```python
from build123d import *

# Parameters (mm, degrees)
F1_DEPTH = 25.4


with BuildPart() as f1:
    # F0 (on Front) → F1 (new body)
    with BuildSketch(Plane.XZ):
        with BuildLine():
            add(Edge.make_bspline(
                [(-41.275, 9.525), (-11.0804249201, 30.3606307657), (19.1141501598, 51.1962615313), (42.965290813, 58.9149246625)],
                knots=[0, 0, 0, 0, 0.5181088639, 0.5181088639, 0.5181088639, 0.5181088639], degree=3))
            Line((-41.275, 9.525), (22.225, 9.525))
            Line((22.225, 9.525), (22.225, 27.0002))
            ThreePointArc((22.225, 27.0002), (27.86556221, 46.0311571047), (42.965290813, 58.9149246625))
        make_face()
        Polygon((22.225, 9.525), (-41.275, 9.525), (-41.275, -9.525), (41.275, -9.525), (41.275, 9.525), align=None)
        with BuildLine():
            Line((22.225, 27.0002), (22.225, 9.525))
            Line((22.225, 9.525), (41.275, 9.525))
            Line((41.275, 9.525), (41.275, 27.0002))
            ThreePointArc((41.275, 27.0002), (45.9246798487, 38.2255201513), (57.15, 42.8752))
            Line((57.15, 42.8752), (60.325, 42.8752))
            Line((60.325, 42.8752), (60.325, 61.9252))
            Line((60.325, 61.9252), (57.15, 61.9252))
            add(Edge.make_bspline(
                [(42.965290813, 58.9149246625), (47.9955126784, 60.5427959923), (52.7435843005, 61.5872364295), (57.15, 61.9252)],
                knots=[0.5181088639, 0.5181088639, 0.5181088639, 0.5181088639, 0.6273783774, 0.6273783774, 0.6273783774, 0.6273783774], degree=3))
            ThreePointArc((42.965290813, 58.9149246625), (27.86556221, 46.0311571047), (22.225, 27.0002))
        make_face()
        with BuildLine():
            ThreePointArc((57.15, 61.9252), (49.8996942767, 61.1643433658), (42.965290813, 58.9149246625))
            add(Edge.make_bspline(
                [(42.965290813, 58.9149246625), (47.9955126784, 60.5427959923), (52.7435843005, 61.5872364295), (57.15, 61.9252)],
                knots=[0.5181088639, 0.5181088639, 0.5181088639, 0.5181088639, 0.6273783774, 0.6273783774, 0.6273783774, 0.6273783774], degree=3))
        make_face()
        with BuildLine():
            add(Edge.make_bspline(
                [(57.15, 61.9252), (58.2283036755, 62.0079038085), (59.2861476071, 62.0483009137), (60.325, 62.0494272736)],
                knots=[0.6273783774, 0.6273783774, 0.6273783774, 0.6273783774, 0.6541179604, 0.6541179604, 0.6541179604, 0.6541179604], degree=3))
            Line((57.15, 61.9252), (60.325, 61.9252))
            Line((60.325, 61.9252), (60.325, 62.0494272736))
        make_face()
        with BuildLine():
            Line((63.5542024739, 61.9252), (60.325, 61.9252))
            Line((60.325, 61.9252), (60.325, 42.8752))
            Line((60.325, 42.8752), (79.5137885917, 42.8752))
            Line((79.5137885917, 42.8752), (79.5137885917, 57.5008483247))
            add(Edge.make_bspline(
                [(63.5542024739, 61.9252), (69.3669017095, 61.4695059449), (74.5907566053, 59.7961982711), (79.5137885917, 57.5008483247)],
                knots=[0.6823542793, 0.6823542793, 0.6823542793, 0.6823542793, 0.8377243298, 0.8377243298, 0.8377243298, 0.8377243298], degree=3))
        make_face()
        with BuildLine():
            Line((60.325, 62.0494272736), (60.325, 61.9252))
            Line((60.325, 61.9252), (63.5542024739, 61.9252))
            add(Edge.make_bspline(
                [(60.325, 62.0494272736), (61.4220016822, 62.050616681), (62.4978262371, 62.0080159778), (63.5542024739, 61.9252)],
                knots=[0.6541179604, 0.6541179604, 0.6541179604, 0.6541179604, 0.6823542793, 0.6823542793, 0.6823542793, 0.6823542793], degree=3))
        make_face()
        with BuildLine():
            Line((60.325, 66.675), (60.325, 62.0494272736))
            add(Edge.make_bspline(
                [(60.325, 62.0494272736), (61.4220016822, 62.050616681), (62.4978262371, 62.0080159778), (63.5542024739, 61.9252)],
                knots=[0.6541179604, 0.6541179604, 0.6541179604, 0.6541179604, 0.6823542793, 0.6823542793, 0.6823542793, 0.6823542793], degree=3))
            Line((63.5542024739, 61.9252), (79.5137885917, 61.9252))
            Line((79.5137885917, 61.9252), (79.5137885917, 57.5008483247))
            Line((79.5137885917, 57.5008483247), (79.5137885917, 42.8752))
            Line((79.5137885917, 42.8752), (60.325, 42.8752))
            Line((60.325, 42.8752), (60.325, 38.1))
            Line((60.325, 38.1), (111.125, 38.1))
            Line((111.125, 38.1), (111.125, 66.675))
            Line((111.125, 66.675), (60.325, 66.675))
        make_face()
    extrude(amount=F1_DEPTH)


solid = f1.part
```
Input: part model. Units: mm. Frame: model coordinates. A direction names the side the tool comes from. Coordinates: 2 decimals unless noted, no trailing zeros. Loops run counter-clockwise (first coordinate to the right, second up) from the corner with the lowest first, then second, coordinate; pieces in that order, holes last. Notation, with made-up numbers: M 20.5,39.25 L 27.5,39.25 A21 ccw 27.5,73.25 Z; hole C 80.5,63.5 d4. An arc over 180 degrees is marked long. Use a Markdown table: item, result. Add a question column.
1) Section A-A, the plane z = -3.5. Return the cut outline in (x, y) (3 decimals).
2) Set-up query: faces 4 (the flat face through (85, -13, 38.1)), 5 (the flat face through (36, 0, 29)), 6 (the flat face through (59, -13, 42.875)), 7 (the flat face through (60.325, -13, 64)). Return all of +Z, -Z, +X, -X, +Y, -Y with unobstructed straight access to the full face (end or side cutting, diameter ignored); none if empty.
3) Section B-B, the plane x = 95.5. Return the cut outline in (y, z) (3 decimals), plus the area to 3 significant figures.
4) Draft query along X for faces 1 (the flat face through (60.325, -13, 41)), 2 (the flat face through (-41.275, -13, 0)), 3 (the flat face through (111.125, -13, 52)). Return one class per face: +X half, -X half, draft (parallel to the pull), parting line (faces both ways), or undercut.
5) Line query: L1, parallel to Z at x = 62.5, y = -23.75 (3 decimals); L2, parallel to X at y = -23, z = -4.5 (3 decimals); L3, parallel to Z at x = 66, y = -6.5 (3 decimals). Output: solid intervals per line, ascending. Write a range as from..to.
6) Pin query (flat end, axial travel): P1, Ø2, axis at y = -12, z = 25, coming from the +X side (3 decimals); P2, Ø5, axis at y = -14, z = 65.5, coming from the -X side (3 decimals); P3, Ø3.5, axis at x = 58.5, y = -11.5, coming from the -Z side. Return the tip coordinate at first contact, or that it passes through.
Answer below:
| question | item | result |
|---|---|---|
| 1 | outline | M -41.275,-25.4 L 41.275,-25.4 L 41.275,0 L -41.275,0 Z |
| 2 | face 4 | -Z, +X, +Y, -Y |
| 2 | face 5 | +Z, -Z, +X, -X, +Y |
| 2 | face 6 | -Z, +Y, -Y |
| 2 | face 7 | +Z, -X, +Y, -Y |
| 3 | outline | M -25.4,38.1 L 0,38.1 L 0,66.675 L -25.4,66.675 Z |
| 3 | area | 726 mm2 |
| 4 | face 1 | undercut |
| 4 | face 2 | -X half |
| 4 | face 3 | +X half |
| 5 | L1 | 38.1..66.675 |
| 5 | L2 | -41.275..41.275 |
| 5 | L3 | 38.1..61.659, 61.925..66.675 |
| 6 | P1 | x = 41.275 |
| 6 | P2 | x = 60.325 |
| 6 | P3 | z = 42.87 |
